from build123d import *

# Parameters (mm, degrees)
SKETCH1_W           = 187
SKETCH1_H           = 262.5
BOSS_EXTRUDE1_DEPTH = 5
SKETCH2_R           = 5
SKETCH2_W           = 100
SKETCH2_H           = 5
CUT_EXTRUDE1_DEPTH  = 5
BOSS_EXTRUDE2_DEPTH = 5
SKETCH3_R           = 2.1
CUT_EXTRUDE2_DEPTH  = 5
CUT_EXTRUDE3_DEPTH  = 2
CUT_EXTRUDE4_DEPTH  = 6
SKETCH8_R           = 2.1
SKETCH8_W           = 5
SKETCH8_H           = 20
CUT_EXTRUDE5_DEPTH  = 10


with BuildPart() as part:
    # Sketch1 → Boss-Extrude1 (new body)
    with BuildSketch(Plane.XY):
        Rectangle(SKETCH1_W, SKETCH1_H)
    extrude(amount=BOSS_EXTRUDE1_DEPTH)

    # Sketch2 → Cut-Extrude1 (cut)
    with BuildSketch(Plane.XY.offset(5)):
        with Locations((0, 133.75)):
            Circle(SKETCH2_R)
        with Locations((0, -128.75)):
            Rectangle(SKETCH2_W, SKETCH2_H)
    extrude(amount=-CUT_EXTRUDE1_DEPTH, mode=Mode.SUBTRACT)

    # Sketch4 → Boss-Extrude2 (add)
    with BuildSketch(Plane.XY.offset(5)):
        with BuildLine():
            Line((33.915063509, 136.25), (44.584936491, 136.25))
            ThreePointArc((44.584936491, 136.25), (48.915063509, 138.75), (53.245190528, 136.25))
            Line((53.245190528, 136.25), (63.915063509, 136.25))
            Line((63.915063509, 136.25), (63.915063509, 131.25))
            Line((63.915063509, 131.25), (33.915063509, 131.25))
            Line((33.915063509, 131.25), (33.915063509, 136.25))
        make_face()
        with BuildLine():
            Line((-53.245190528, 136.25), (-63.915063509, 136.25))
            Line((-63.915063509, 136.25), (-63.915063509, 131.25))
            Line((-63.915063509, 131.25), (-33.915063509, 131.25))
            Line((-33.915063509, 131.25), (-33.915063509, 136.25))
            Line((-33.915063509, 136.25), (-44.584936491, 136.25))
            ThreePointArc((-44.584936491, 136.25), (-48.915063509, 138.75), (-53.245190528, 136.25))
        make_face()
    extrude(amount=-BOSS_EXTRUDE2_DEPTH)

    # Sketch3 → Cut-Extrude2 (cut)
    with BuildSketch(Plane.XY.offset(5)):
        with Locations((-48.915063509, 133.75)):
            Circle(SKETCH3_R)
        with Locations((48.915063509, 133.75)):
            Circle(SKETCH3_R)
        with Locations((-48.915063509, -63.75)):
            Circle(SKETCH3_R)
        with Locations((0, -63.75)):
            Circle(SKETCH3_R)
        with Locations((48.915063509, -63.75)):
            Circle(SKETCH3_R)
        Polygon((-32.90655119, -126.25), (-32.90655119, -116.25), (-30.00655119, -116.25), (-30.00655119, -111.25), (-23.80655119, -111.25), (-23.80655119, -116.25), (-20.90655119, -116.25), (-20.90655119, -126.25), align=None)
        Polygon((32.90655119, -126.25), (20.90655119, -126.25), (20.90655119, -116.25), (23.80655119, -116.25), (23.80655119, -111.25), (30.00655119, -111.25), (30.00655119, -116.25), (32.90655119, -116.25), align=None)
    extrude(amount=-CUT_EXTRUDE2_DEPTH, mode=Mode.SUBTRACT)

    # Sketch5 → Cut-Extrude3 (cut)
    with BuildSketch(Plane.XY.offset(5)):
        with BuildLine():
            Line((-24.33400194, 77.119068048), (24.33400194, 77.119068048))
            ThreePointArc((24.33400194, 77.119068048), (26.453069989, 75), (24.33400194, 72.880931952))
            Line((24.33400194, 72.880931952), (-24.33400194, 72.880931952))
            ThreePointArc((-24.33400194, 72.880931952), (-26.453069989, 75), (-24.33400194, 77.119068048))
        make_face()
        with BuildLine():
            Line((-24.33400194, 67.119068048), (24.33400194, 67.119068048))
            ThreePointArc((24.33400194, 67.119068048), (26.453069989, 65), (24.33400194, 62.880931952))
            Line((24.33400194, 62.880931952), (-24.33400194, 62.880931952))
            ThreePointArc((-24.33400194, 62.880931952), (-26.453069989, 65), (-24.33400194, 67.119068048))
        make_face()
        with BuildLine():
            Line((-24.33400194, 57.119068048), (24.33400194, 57.119068048))
            ThreePointArc((24.33400194, 57.119068048), (26.453069989, 55), (24.33400194, 52.880931952))
            Line((24.33400194, 52.880931952), (-24.33400194, 52.880931952))
            ThreePointArc((-24.33400194, 52.880931952), (-26.453069989, 55), (-24.33400194, 57.119068048))
        make_face()
        with BuildLine():
            Line((-24.33400194, 47.119068048), (24.33400194, 47.119068048))
            ThreePointArc((24.33400194, 47.119068048), (26.453069989, 45), (24.33400194, 42.880931952))
            Line((24.33400194, 42.880931952), (-24.33400194, 42.880931952))
            ThreePointArc((-24.33400194, 42.880931952), (-26.453069989, 45), (-24.33400194, 47.119068048))
        make_face()
        with BuildLine():
            Line((-24.33400194, 37.119068048), (24.33400194, 37.119068048))
            ThreePointArc((24.33400194, 37.119068048), (26.453069989, 35), (24.33400194, 32.880931952))
            Line((24.33400194, 32.880931952), (-24.33400194, 32.880931952))
            ThreePointArc((-24.33400194, 32.880931952), (-26.453069989, 35), (-24.33400194, 37.119068048))
        make_face()
        with BuildLine():
            Line((-24.33400194, 27.119068048), (24.33400194, 27.119068048))
            ThreePointArc((24.33400194, 27.119068048), (26.453069989, 25), (24.33400194, 22.880931952))
            Line((24.33400194, 22.880931952), (-24.33400194, 22.880931952))
            ThreePointArc((-24.33400194, 22.880931952), (-26.453069989, 25), (-24.33400194, 27.119068048))
        make_face()
        with BuildLine():
            Line((78.954073016, -17.485670168), (54.620071076, -59.63339788))
            ThreePointArc((54.620071076, -59.63339788), (51.72537029, -60.409030618), (50.949737551, -57.514329832))
            Line((50.949737551, -57.514329832), (75.283739492, -15.36660212))
            ThreePointArc((75.283739492, -15.36660212), (78.178440278, -14.590969382), (78.954073016, -17.485670168))
        make_face()
        with BuildLine():
            Line((70.293818978, -12.485670168), (45.959817038, -54.63339788))
            ThreePointArc((45.959817038, -54.63339788), (43.065116252, -55.409030618), (42.289483514, -52.514329832))
            Line((42.289483514, -52.514329832), (66.623485454, -10.36660212))
            ThreePointArc((66.623485454, -10.36660212), (69.51818624, -9.590969382), (70.293818978, -12.485670168))
        make_face()
        with BuildLine():
            Line((61.633564941, -7.485670168), (37.299563, -49.63339788))
            ThreePointArc((37.299563, -49.63339788), (34.404862214, -50.409030618), (33.629229476, -47.514329832))
            Line((33.629229476, -47.514329832), (57.963231416, -5.36660212))
            ThreePointArc((57.963231416, -5.36660212), (60.857932202, -4.590969382), (61.633564941, -7.485670168))
        make_face()
        with BuildLine():
            Line((52.973310903, -2.485670168), (28.639308963, -44.63339788))
            ThreePointArc((28.639308963, -44.63339788), (25.744608176, -45.409030618), (24.968975438, -42.514329832))
            Line((24.968975438, -42.514329832), (49.302977378, -0.36660212))
            ThreePointArc((49.302977378, -0.36660212), (52.197678165, 0.409030618), (52.973310903, -2.485670168))
        make_face()
        with BuildLine():
            Line((44.313056865, 2.514329832), (19.979054925, -39.63339788))
            ThreePointArc((19.979054925, -39.63339788), (17.084354138, -40.409030618), (16.3087214, -37.514329832))
            Line((16.3087214, -37.514329832), (40.64272334, 4.63339788))
            ThreePointArc((40.64272334, 4.63339788), (43.537424127, 5.409030618), (44.313056865, 2.514329832))
        make_face()
        with BuildLine():
            Line((35.652802827, 7.514329832), (11.318800887, -34.63339788))
            ThreePointArc((11.318800887, -34.63339788), (8.4241001, -35.409030618), (7.648467362, -32.514329832))
            Line((7.648467362, -32.514329832), (31.982469302, 9.63339788))
            ThreePointArc((31.982469302, 9.63339788), (34.877170089, 10.409030618), (35.652802827, 7.514329832))
        make_face()
        with BuildLine():
            Line((-54.620071076, -59.63339788), (-78.954073016, -17.485670168))
            ThreePointArc((-78.954073016, -17.485670168), (-78.178440278, -14.590969382), (-75.283739492, -15.36660212))
            Line((-75.283739492, -15.36660212), (-50.949737551, -57.514329832))
            ThreePointArc((-50.949737551, -57.514329832), (-51.72537029, -60.409030618), (-54.620071076, -59.63339788))
        make_face()
        with BuildLine():
            Line((-45.959817038, -54.63339788), (-70.293818978, -12.485670168))
            ThreePointArc((-70.293818978, -12.485670168), (-69.51818624, -9.590969382), (-66.623485454, -10.36660212))
            Line((-66.623485454, -10.36660212), (-42.289483514, -52.514329832))
            ThreePointArc((-42.289483514, -52.514329832), (-43.065116252, -55.409030618), (-45.959817038, -54.63339788))
        make_face()
        with BuildLine():
            Line((-37.299563, -49.63339788), (-61.633564941, -7.485670168))
            ThreePointArc((-61.633564941, -7.485670168), (-60.857932202, -4.590969382), (-57.963231416, -5.36660212))
            Line((-57.963231416, -5.36660212), (-33.629229476, -47.514329832))
            ThreePointArc((-33.629229476, -47.514329832), (-34.404862214, -50.409030618), (-37.299563, -49.63339788))
        make_face()
        with BuildLine():
            Line((-28.639308963, -44.63339788), (-52.973310903, -2.485670168))
            ThreePointArc((-52.973310903, -2.485670168), (-52.197678165, 0.409030618), (-49.302977378, -0.36660212))
            Line((-49.302977378, -0.36660212), (-24.968975438, -42.514329832))
            ThreePointArc((-24.968975438, -42.514329832), (-25.744608176, -45.409030618), (-28.639308963, -44.63339788))
        make_face()
        with BuildLine():
            Line((-19.979054925, -39.63339788), (-44.313056865, 2.514329832))
            ThreePointArc((-44.313056865, 2.514329832), (-43.537424127, 5.409030618), (-40.64272334, 4.63339788))
            Line((-40.64272334, 4.63339788), (-16.3087214, -37.514329832))
            ThreePointArc((-16.3087214, -37.514329832), (-17.084354138, -40.409030618), (-19.979054925, -39.63339788))
        make_face()
        with BuildLine():
            Line((-11.318800887, -34.63339788), (-35.652802827, 7.514329832))
            ThreePointArc((-35.652802827, 7.514329832), (-34.877170089, 10.409030618), (-31.982469302, 9.63339788))
            Line((-31.982469302, 9.63339788), (-7.648467362, -32.514329832))
            ThreePointArc((-7.648467362, -32.514329832), (-8.4241001, -35.409030618), (-11.318800887, -34.63339788))
        make_face()
    extrude(amount=-CUT_EXTRUDE3_DEPTH, mode=Mode.SUBTRACT)

    # Sketch6 → Cut-Extrude4 (cut, through all)
    with BuildSketch(Plane.XY.offset(5)):
        Polygon((-24.33400194, 32.880931952), (24.33400194, 32.880931952), (40.64272334, 4.63339788), (16.3087214, -37.514329832), (-16.3087214, -37.514329832), (-40.64272334, 4.63339788), align=None)
    extrude(amount=-CUT_EXTRUDE4_DEPTH, mode=Mode.SUBTRACT)

    # Sketch8 → Cut-Extrude5 (cut)
    with BuildSketch(Plane.XY.offset(5)):
        with Locations((0, -47.514329832)):
            Circle(SKETCH8_R)
        with Locations((-41.148616678, 23.757164916)):
            Circle(SKETCH8_R)
        with Locations((41.148616678, 23.757164916)):
            Circle(SKETCH8_R)
        with Locations((-26.806655169, 103.979066034)):
            Rectangle(SKETCH8_W, SKETCH8_H)
        with Locations((26.806655169, 103.979066034)):
            Rectangle(SKETCH8_W, SKETCH8_H)
    extrude(amount=-CUT_EXTRUDE5_DEPTH, mode=Mode.SUBTRACT)


solid = part.part
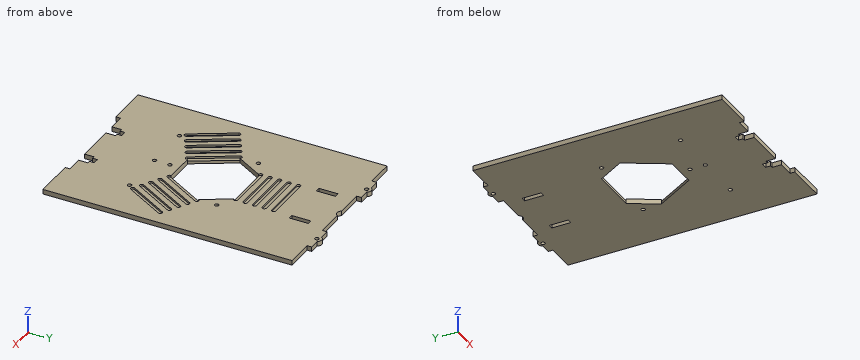
Input: part model. Units: mm. Frame: model coordinates. Coordinates: 2 decimals unless noted, no trailing zeros.
(1) First-contact query: pin 1 Ø1 at (x, z) = (4.5, 4) entering from -Y; pin 2 Ø1 at (x, z) = (11, 4) entering from +Y; pin 3 Ø1.5 at (x, z) = (-22, 3) entering from -Y. Flat tips, straight axial feed; report the tip coordinate or a pass-through.
(2) Section A-A on z = 3.9. Count the separate pieces of the cut face and the enclosed holes in it, then the cut area to 3 significant figures.
(3) Material intervals for probe 1 along X at (y, z) = (112.5, 2.95); probe 2 along Y at (x, z) = (13, 1.7); probe 3 along X at (y, z) = (133.75, 3.85), sorted ascending.
Data:
1. pin 1: stops at y = -126.25
1. pin 2: stops at y = 131.25
1. pin 3: stops at y = -116.25
2. separate pieces: 1
2. enclosed holes: 23
2. area: 40,700 mm2
3. probe 1: x = -93.5 to -29.31, -24.31 to 24.31, 29.31 to 93.5
3. probe 2: y = -126.25 to -37.51, 32.88 to 131.25
3. probe 3: x = -63.92 to -51.02, -46.82 to -33.92, 33.92 to 46.82, 51.02 to 63.92
